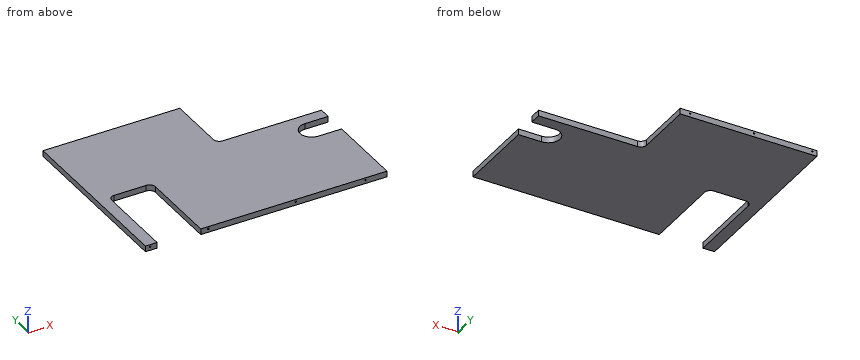
Autodesk Inventor part; units mm, degrees
ref_plane "YZ Plane" through (0, 0, 0) normal (1, 0, 0) x (0, 1, 0)
ref_plane "XZ Plane" through (0, 0, 0) normal (0, 1, 0) x (-1, 0, 0)
ref_plane "XY Plane" through (0, 0, 0) normal (0, 0, 1) x (1, 0, 0)
sketch "Sketch1" plane through (0, 0, 0) normal (0, 0, 1) x (1, 0, 0)
  line L0 (-207.5, -152.5) -> (207.5, -152.5)
  line L1 (207.5, -152.5) -> (207.5, 152.5)
  line L2 (207.5, 152.5) -> (-207.5, 152.5)
  line L3 (-207.5, 152.5) -> (-207.5, -152.5)
  line L4 (-207.5, -152.5) -> (207.5, 152.5) construction
  line L5 (207.5, -152.5) -> (-207.5, 152.5) construction
  point P0 (0, 0)
  dimension "d0" = 415
  dimension "d1" = 305
extrude "Extrusion1" add sketch "Sketch1" along normal blind 10
sketch "Sketch2" plane through (0, 0, 10) normal (0, 0, 1) x (1, 0, 0)
  line L0 (-207.5, -152.5) -> (207.5, -152.5)
  line L1 (-187.5, -152.5) -> (-112.5, -152.5)
  line L2 (-112.5, -152.5) -> (-112.5, -17.5)
  line L3 (-122.5, -7.5) -> (-177.5, -7.5)
  line L4 (-187.5, -17.5) -> (-187.5, -152.5)
  line L5 (-207.5, 152.5) -> (-207.5, -152.5)
  line L6 (207.5, -152.5) -> (207.5, 152.5)
  line L7 (207.5, 22.5) -> (167.5, 22.5)
  line L8 (167.5, 22.5) -> (167.5, -17.5) construction
  line L9 (167.5, -17.5) -> (207.5, -17.5)
  line L10 (207.5, -17.5) -> (207.5, 22.5)
  line L11 (207.5, 152.5) -> (-207.5, 152.5)
  arc A0 (167.5, 22.5) -> (167.5, -17.5) centre (167.5, 2.5) ccw
  line L12 (27.5, 152.5) -> (207.5, 152.5)
  line L13 (207.5, 152.5) -> (207.5, 42.5)
  line L14 (207.5, 42.5) -> (37.5, 42.5)
  line L15 (27.5, 52.5) -> (27.5, 152.5)
  arc A1 (-177.5, -7.5) -> (-187.5, -17.5) centre (-177.5, -17.5) ccw
  arc A2 (-112.5, -17.5) -> (-122.5, -7.5) centre (-122.5, -17.5) ccw
  arc A3 (27.5, 52.5) -> (37.5, 42.5) centre (37.5, 52.5) ccw
  point P0 (0, 0)
  point P1 (-112.5, -7.5)
  point P2 (-187.5, -7.5)
  point P3 (27.5, 42.5)
  dimension "d4" = 145
  dimension "d5" = 75
  dimension "d6" = 20
  dimension "d7" = 40
  dimension "d8" = 40
  dimension "d9" = 130
  dimension "d10" = 110
  dimension "d11" = 180
  dimension "d41" = 10
extrude "Extrusion2" cut sketch "Sketch2" against normal blind 10 contours L4 A1 L3 A2 L2 L0 | L11 L6 L14 A3 L15 | L9 A0 L7 L6
sketch "Sketch3" plane through (207.5, -152.5, 0) normal (0, -1, 0) x (1, 0, 0)
  line L0 (-415, 0) -> (-415, 10)
  line L1 (-415, 6) -> (0, 6) construction
  line L2 (0, 10) -> (0, 0)
  line L3 (-320, 0) -> (0, 0) construction
  line L4 (-395, 0) -> (-395, 10) construction
  point P0 (-207.5, 0)
  point P1 (-407, 6)
  point P2 (-307, 6)
  point P3 (-37, 6)
  point P4 (-157, 6)
  dimension "d14" = 6
  dimension "d15" = 415
  dimension "d16" = 20
  dimension "d17" = 8
  dimension "d18" = 100
  dimension "d19" = 150
  dimension "d20" = 120
sketch "Sketch4" plane through (-207.5, 152.5, 10) normal (0, 1, 0) x (1, 0, 0)
  line L0 (0, 10) -> (0, 0)
  line L1 (0, 4) -> (235, 4) construction
  line L2 (235, 10) -> (0, 10)
  point P0 (207.5, 10)
  point P1 (8, 4)
  point P2 (108, 4)
  point P3 (218, 4)
  dimension "d22" = 6
  dimension "d23" = 8
  dimension "d24" = 210
  dimension "d25" = 100
hole "Hole1" at (-199.5, -152.5, 6) at (-99.5, -152.5, 6) at (50.5, -152.5, 6) at (170.5, -152.5, 6) direction (0, 1, 0) diameter 2.459 depth 10
hole "Hole2" at (10.5, 152.5, 6) at (-99.5, 152.5, 6) at (-199.5, 152.5, 6) direction (0, -1, 0) diameter 2.459 depth 10
properties part number "Bottom"
Input: part model. Units: mm. Frame: model coordinates. Coordinates: 2 decimals unless noted, no trailing zeros. Loops run counter-clockwise (first coordinate to the right, second up) from the corner with the lowest first, then second, coordinate; pieces in that order, holes last. Notation, with made-up numbers: (44.5, 80.25) - (82.5, 80.25) arc R22 ccw to (82.5, 113.25) - close; hole circle Ø11 at (-20, 69.25). An arc over 180 degrees is marked (long way). Answer in a Markdown table with one row per item. Add a question column.
Item 1: Line query: line 1 along X through (y, z) = (-145, 6); line 2 along X through (y, z) = (-123.5, 1.75); line 3 along X through (y, z) = (149, 6). Output: solid intervals per line, ascending. Write a range as [from, to].
Item 2: Section query A-A on y = -77. Return the cut outline in (x, z).
Item 3: Section query D-D on y = 2.5. Return the cut outline in (x, z), then the cut area to 3 significant figures.
Item 4: Section query B-B on z = 1.75. Return the cut outline in (x, y), then the cut area to 3 significant figures.
Item 5: Section query C-C on x = -139.5. Return the cut outline in (y, z).
Item 6: Contact query for flat-ended pins moving along their axis: P1, Ø3, axis at x = 182.5, z = 3.5, coming from the +Y side; P2, Ø2, axis at x = -99.5, z = 6, coming from the +Y side; P3, Ø0.7, axis at x = -199, z = 6.5, coming from the -Y side. Output: stop coordinate, or through.
Recorded:
| question | item | result |
|---|---|---|
| 1 | line 1 | [-207.5, -200.73], [-198.27, -187.5], [-112.5, -100.73], [-98.27, 49.27], [51.73, 169.27], [171.73, 207.5] |
| 1 | line 2 | [-207.5, -187.5], [-112.5, 207.5] |
| 1 | line 3 | [-207.5, -200.73], [-198.27, -100.73], [-98.27, 9.27], [11.73, 27.5] |
| 2 | outline | (-207.5, 0) - (-187.5, 0) - (-187.5, 10) - (-207.5, 10) - close; (-112.5, 0) - (207.5, 0) - (207.5, 10) - (-112.5, 10) - close |
| 3 | outline | (-207.5, 0) - (147.5, 0) - (147.5, 10) - (-207.5, 10) - close |
| 3 | area | 3,550 mm^2 |
| 4 | outline | (-207.5, -152.5) - (-187.5, -152.5) - (-187.5, -17.5) arc R10 cw to (-177.5, -7.5) - (-122.5, -7.5) arc R10 cw to (-112.5, -17.5) - (-112.5, -152.5) - (207.5, -152.5) - (207.5, -17.5) - (167.5, -17.5) arc R20 cw to (167.5, 22.5) - (207.5, 22.5) - (207.5, 42.5) - (37.5, 42.5) arc R10 cw to (27.5, 52.5) - (27.5, 152.5) - (-207.5, 152.5) - close |
| 4 | area | 93,700 mm^2 |
| 5 | outline | (-7.5, 0) - (152.5, 0) - (152.5, 10) - (-7.5, 10) - close |
| 6 | P1 | y = 42.5 |
| 6 | P2 | y = 142.5 |
| 6 | P3 | y = -142.5 |
